from build123d import *

# Parameters (mm, degrees)
SKETCH1_W           = 40
SKETCH1_H           = 60
BOSS_EXTRUDE4_DEPTH = 3
SKETCH5_W           = 15
SKETCH5_H           = 25
CUT_EXTRUDE2_DEPTH  = 1
SKETCH7_R           = 1
CUT_EXTRUDE3_DEPTH  = 2
SKETCH8_R           = 1
CUT_EXTRUDE4_DEPTH  = 2
FILLET1_R           = 5
SKETCH12_R          = 1
CUT_EXTRUDE6_DEPTH  = 12
SKETCH13_W          = 15
SKETCH13_H          = 25
CUT_EXTRUDE7_DEPTH  = 1
SKETCH14_R          = 1
CUT_EXTRUDE8_DEPTH  = 7


with BuildPart() as part:
    # Sketch1 → Boss-Extrude4 (new body)
    with BuildSketch(Plane.XY):
        with Locations((-45.9850693, -3.193565597)):
            Rectangle(SKETCH1_W, SKETCH1_H)
    extrude(amount=-BOSS_EXTRUDE4_DEPTH)

    # Sketch5 → Cut-Extrude2 (cut)
    with BuildSketch(Plane.XY):
        with Locations((-58.4850693, -3.193565597)):
            Rectangle(SKETCH5_W, SKETCH5_H)
    extrude(amount=-CUT_EXTRUDE2_DEPTH, mode=Mode.SUBTRACT)

    # Sketch7 → Cut-Extrude3 (cut)
    with BuildSketch(Plane.XY.offset(-1)):
        with Locations((-55.9850693, 4.306434403)):
            Circle(SKETCH7_R)
    extrude(amount=-CUT_EXTRUDE3_DEPTH, mode=Mode.SUBTRACT)

    # Sketch8 → Cut-Extrude4 (cut)
    with BuildSketch(Plane.XY.offset(-1)):
        with Locations((-55.9850693, -10.693565597)):
            Circle(SKETCH8_R)
    extrude(amount=-CUT_EXTRUDE4_DEPTH, mode=Mode.SUBTRACT)

    # Fillet1
    fillet1_edges = [part.edges().sort_by_distance(p)[0] for p in [
        (-65.9850693, 26.806434403, -1.5),
        (-65.9850693, -33.193565597, -1.5),
        (-25.9850693, -33.193565597, -1.5),
        (-25.9850693, 26.806434403, -1.5),
    ]]
    fillet(fillet1_edges, radius=FILLET1_R)

    # Sketch12 → Cut-Extrude6 (cut)
    with BuildSketch(Plane(origin=(0, 0, -3), x_dir=(-1, 0, 0), z_dir=(0, 0, -1))):
        with Locations((45.9850693, -3.193565597)):
            Circle(SKETCH12_R)
    extrude(amount=-CUT_EXTRUDE6_DEPTH, mode=Mode.SUBTRACT)

    # Sketch13 → Cut-Extrude7 (cut)
    with BuildSketch(Plane.XY):
        with Locations((-33.4850693, -3.4366123)):
            Rectangle(SKETCH13_W, SKETCH13_H)
    extrude(amount=-CUT_EXTRUDE7_DEPTH, mode=Mode.SUBTRACT)

    # Sketch14 → Cut-Extrude8 (cut)
    with BuildSketch(Plane.XY.offset(-1)):
        with Locations((-35.9850693, 4.0633877)):
            Circle(SKETCH14_R)
        with Locations((-35.9850693, -10.9366123)):
            Circle(SKETCH14_R)
    extrude(amount=-CUT_EXTRUDE8_DEPTH, mode=Mode.SUBTRACT)


solid = part.part
Input: part model. Units: mm. Frame: model coordinates. A direction names the side the tool comes from. Coordinates: 2 decimals unless noted, no trailing zeros. Loops run counter-clockwise (first coordinate to the right, second up) from the corner with the lowest first, then second, coordinate; pieces in that order, holes last. Notation, with made-up numbers: (75, 87) -> (93, 87) arc R19 cw to (93, 121) -> close; hole circle Ø6 at (-19.5, 3.5). An arc over 180 degrees is marked (long way). Write each question's results on one line, items separated by ' | '. Start each with the question number.
Q1. Ray query, line 1 (Y direction, x = -57.5, z = -0.85); line 2 (Y direction, x = -35.5, z = -2.6); line 3 (Z direction, x = -55, y = 3). Return the intervals inside material, ascending. Write a range as from..to.
Q2. Pin query (flat end, axial travel): pin 1 (2.5 mm diameter, centred on x = -45.99, y = -3.19, fed in from -Z); pin 2 (4.5 mm diameter, centred on x = -58.5, y = -2, fed in from +Z); pin 3 (0.8 mm diameter, centred on y = 2.5, z = -0.5, fed in from +X); pin 4 (0.8 mm diameter, centred on y = -1, z = -0.5, fed in from -X). Return the tip coordinate at first contact, or that it passes through.
Q3. Section D-D, the plane x = -63. Return the cut outline in (y, z), plus the area to 3 significant figures.
Q4. Reachability of faces 4 (the flat face through (-59, -3, -1)), 5 (the flat face through (-46, 26.806, -1)), 6 (the flat face through (-34, -3, -1)) from +Z, -Z, +X, -X, +Y, -Y: full face, straight path, thin tool, end or side. Return the list, or none.
Q5. Section C-C, the plane z = -1.7. Return the cut outline in (x, y).
Q6. Section B-B, the plane x = -46. Return the cut outline in (y, z).
Q7. Pull-direction query (Y, two-part tool) for faces 1 (the cylindrical face through (-64.56, -31.69, -1.52)), 2 (the cylindrical face through (-27.49, 25.38, -1.52)), 3 (the cylindrical face through (-36.984, -10.893, -1.986)); classes: released by +Y, released by -Y, zero draft, split by the parting line, or undercut.
Q8. Section A-A, the plane y = 1.5. Return the cut outline in (x, z).
Found:
1) line 1: -33.19..-15.69, 9.31..26.81 | line 2: -33.19..-11.81, -10.06..3.19, 4.94..26.81 | line 3: -3..-1
2) pin 1: z = -3 | pin 2: z = -1 | pin 3: x = -40.99 | pin 4: x = -50.99
3) outline: (-32.77, -3) -> (26.38, -3) -> (26.38, 0) -> (9.31, 0) -> (9.31, -1) -> (-15.69, -1) -> (-15.69, 0) -> (-32.77, 0) -> close | area: 152 mm2
4) face 4: +Z, -X | face 5: +Z, -Z, +X, -X, +Y | face 6: +Z, +X
5) outline: (-65.99, -28.19) arc R5 ccw to (-60.99, -33.19) -> (-30.99, -33.19) arc R5 ccw to (-25.99, -28.19) -> (-25.99, 21.81) arc R5 ccw to (-30.99, 26.81) -> (-60.99, 26.81) arc R5 ccw to (-65.99, 21.81) -> close; hole circle Ø2 at (-55.99, -10.69); hole circle Ø2 at (-55.99, 4.31); hole circle Ø2 at (-45.99, -3.19); hole circle Ø2 at (-35.99, -10.94); hole circle Ø2 at (-35.99, 4.06)
6) outline: (-33.19, -3) -> (-4.19, -3) -> (-4.19, 0) -> (-33.19, 0) -> close; (-2.19, -3) -> (26.81, -3) -> (26.81, 0) -> (-2.19, 0) -> close
7) face 1: released by -Y | face 2: released by +Y | face 3: undercut
8) outline: (-65.99, -3) -> (-25.99, -3) -> (-25.99, -1) -> (-40.99, -1) -> (-40.99, 0) -> (-50.99, 0) -> (-50.99, -1) -> (-65.99, -1) -> close
